Geometry check sheet. Reference: the model listing, model coordinates, mm. A direction names the side the tool comes from. Round coordinates to 2 decimals unless told otherwise and drop trailing zeros. Order: outer loops, then holes, each group sorted by start corner. A loop starts at its lowest first (then second) coordinate and runs counter-clockwise, first axis right, second up.
(1) Draft check along X on faces 1 (the face through (1.571, -13.675, 5.156)), 2 (the face through (36.842, -22, 17)), 3 (the face through (5, -25, 0)). Enter one of: pulls with the +X half, pulls with the -X half, needs draft (parallel to the pull), parting line crosses it, or undercut.
(2) Gauge pin test, flat ends, axial feed: P1, Ø8, axis at y = -8.5, z = 7.5, coming from the -X side; P2, Ø1, axis at x = -34.5, z = 5, coming from the +Y side; P3, Ø8, axis at x = 4.5, y = -27, coming from the +Z side; P4, Ø8, axis at x = 10, z = 14.5, coming from the +Y side. Record the tip position at first contact, or that the pin passes through.
(3) Cross-section at C-C on x = 8. Enter the section's corners in (y, z), and give its area (3 significant figures).
(4) Thickness scan on L1, parallel to X at y = -11, z = 10.5; L2, parallel to Y at x = -45, z = 5.5; L3, parallel to Z at x = -31.5, y = -29. Record the ranges inside material, lowest first.
(5) Cross-section at B-B on z = 8.5. Enter the section's corners in (x, y), and give its area (3 significant figures).
(6) Set-up check for faces 4 (the face through (-43, -19.808, 5)), 5 (the face through (50, -9, 17.028)), 6 (the face through (-8, -17, 10.17)), 7 (the face through (-51.084, -27, 5)): record each of +Z, -Z, +X, -X, +Y, -Y from which the full face is reachable in a straight line by a thin tool's end or side.
(7) Cross-section at A-A on y = -21. Enter the section's corners in (x, z).
(8) Cross-section at D-D on z = 14.5. Enter the section's corners in (x, y).
from build123d import *

# Parameters (mm, degrees)
F0_W     = 114.3
F0_H     = 10.170036
F1_DEPTH = 34.798
F2_W     = 17.233886
F2_H     = 19.807858
F3_DEPTH = 25.4
F4_W     = 26.374524
F4_H     = 34.798
F5_DEPTH = 17.272
F6_W     = 26.374524
F6_H     = 17.399
F7_DEPTH = 10.414
F8_R     = 5.509405
F9_DEPTH = 35.56


with BuildPart() as f1:
    # F0 (on Front) → F1 (new body)
    with BuildSketch(Plane.XZ):
        with Locations((6.0662, 5.085018)):
            Rectangle(F0_W, F0_H)
    extrude(amount=F1_DEPTH)

    # F2 (on face) → F3 (cut)
    with BuildSketch(Plane.XY.offset(10.170036)):
        with Locations((-42.466857, -9.903929)):
            Rectangle(F2_W, F2_H)
    extrude(amount=-F3_DEPTH, mode=Mode.SUBTRACT)

    # F4 (on face) → F5 (join)
    with BuildSketch(Plane.XY.offset(10.170036)):
        with Locations((50.028938, -17.399)):
            Rectangle(F4_W, F4_H)
    extrude(amount=F5_DEPTH)

    # F6 (on face) → F7 (cut)
    with BuildSketch(Plane.XY.offset(27.442036)):
        with Locations((50.028938, -8.6995)):
            Rectangle(F6_W, F6_H)
    extrude(amount=-F7_DEPTH, mode=Mode.SUBTRACT)

    # F8 (on face) → F9 (cut)
    with BuildSketch(Plane.XY.offset(10.170036)):
        with Locations((5.631648, -17.399)):
            Circle(F8_R)
    extrude(amount=-F9_DEPTH, mode=Mode.SUBTRACT)


solid = f1.part
Found:
1. face 1: undercut
1. face 2: pulls with the -X half
1. face 3: needs draft
2. P1: stops at x = -33.85
2. P2: stops at y = -19.81
2. P3: stops at z = 10.17
2. P4: passes through
3. outline: (-34.8, 0) - (-22.37, 0) - (-22.37, 10.17) - (-34.8, 10.17) - close; (-12.42, 0) - (0, 0) - (0, 10.17) - (-12.42, 10.17) - close
3. area: 253 mm2
4. L1: x = 36.84 to 63.22
4. L2: y = -34.8 to -19.81
4. L3: z = 0 to 10.17
5. outline: (-51.08, -34.8) - (63.22, -34.8) - (63.22, 0) - (-33.85, 0) - (-33.85, -19.81) - (-51.08, -19.81) - close; hole circle Ø11.02 at (5.63, -17.4)
5. area: 3,540 mm2
6. face 4: +Z, -Z, -X, +Y
6. face 5: +Z, +X, -X, +Y
6. face 6: +Z, -X, +Y, -Y
6. face 7: +Z, -Z, -X, +Y, -Y
7. outline: (-51.08, 0) - (1.46, 0) - (1.46, 10.17) - (-51.08, 10.17) - close; (9.8, 0) - (63.22, 0) - (63.22, 27.44) - (36.84, 27.44) - (36.84, 10.17) - (9.8, 10.17) - close
8. outline: (36.84, -34.8) - (63.22, -34.8) - (63.22, 0) - (36.84, 0) - close
